Verification items for the finished model (mm, model axes). A direction names the side the tool comes from. Round coordinates to 2 decimals unless told otherwise and drop trailing zeros. Write each loop counter-clockwise with the first axis right and the second up, starting at its lowest first coordinate (ties: lowest second). Pieces come first, ordered by that corner, then holes.
from build123d import *
from build123d.topology import SkipClean

# Parameters (mm, degrees)
CUT_EXTRUDE1_DEPTH      = 35
CUT_EXTRUDE1_DEPTH_BACK = 35
SKETCH2_OUTSIDE_W       = 96.248
SKETCH2_OUTSIDE_H       = 96.248
BOSS_EXTRUDE1_DEPTH     = 36
SKETCH4_R               = 3.5
CUT_EXTRUDE2_DEPTH      = 5
LPATTERN1_COUNT         = 2
LPATTERN1_PITCH         = 35
BOSS_EXTRUDE2_DEPTH     = 50
BOSS_EXTRUDE6_DEPTH     = 15
SKETCH10_R              = 25
BOSS_EXTRUDE7_DEPTH     = 2
SKETCH11_R              = 3.5
BOSS_EXTRUDE8_DEPTH     = 5


with BuildPart() as part:
    # Sketch1 → Revolve2 (revolve)
    with BuildSketch(Plane(origin=(0, 0, 0), x_dir=(1, 0, 0), z_dir=(0, 1, 0))):
        with BuildLine():
            Line((0, 35), (0, -35))
            ThreePointArc((0, -35), (35, 0), (0, 35))
        make_face()
    revolve(axis=Axis((0, 0, -35), (0, 0, 1)))

    # Sketch2 outside → Cut-Extrude1 (cut, two sides: drawn at the far end of the back side and taken through both)
    with SkipClean():  # the faces are left unmerged after this step: merging them gives an invalid solid
        with BuildSketch(Plane(origin=(0, 0, 0), x_dir=(1, 0, 0), z_dir=(0, 1, 0)).offset(-CUT_EXTRUDE1_DEPTH_BACK)):
            Rectangle(SKETCH2_OUTSIDE_W, SKETCH2_OUTSIDE_H)
            with BuildLine():
                Line((-20, -28.722813233), (-20, 28.722813233))
                ThreePointArc((-20, 28.722813233), (0, 35), (20, 28.722813233))
                Line((20, 28.722813233), (20, -28.722813233))
                ThreePointArc((20, -28.722813233), (0, -35), (-20, -28.722813233))
            make_face(mode=Mode.SUBTRACT)
        extrude(amount=CUT_EXTRUDE1_DEPTH + CUT_EXTRUDE1_DEPTH_BACK, mode=Mode.SUBTRACT)

    # Sketch3 → Boss-Extrude1 (add)
    with BuildSketch(Plane(origin=(0, 0, 0), x_dir=(1, 0, 0), z_dir=(0, 1, 0))):
        with BuildLine():
            Line((-20, 15), (-20, -15))
            ThreePointArc((-20, -15), (0, -25), (20, -15))
            Line((20, -15), (20, 15))
            ThreePointArc((20, 15), (0, 25), (-20, 15))
        make_face()
    extrude(amount=BOSS_EXTRUDE1_DEPTH)

    # Sketch4 → Cut-Extrude2 (cut)
    with BuildSketch(Plane.ZY.offset(20)):
        Circle(SKETCH4_R)
    cut_extrude2 = extrude(amount=-CUT_EXTRUDE2_DEPTH, mode=Mode.SUBTRACT)

    # LPattern1: Cut-Extrude2 ×2
    with Locations(*[(i * LPATTERN1_PITCH, 0, 0) for i in range(1, LPATTERN1_COUNT)]):
        add(cut_extrude2, mode=Mode.SUBTRACT)

    # Sketch5 → Boss-Extrude2 (add)
    with BuildSketch(Plane(origin=(0, 36, 0), x_dir=(1, 0, 0), z_dir=(0, 1, 0))):
        with BuildLine():
            Line((-20, 15), (-20, 11.357816692))
            ThreePointArc((-20, 11.357816692), (-23, 0), (-20, -11.357816692))
            Line((-20, -11.357816692), (-20, -15))
            ThreePointArc((-20, -15), (0, -25), (20, -15))
            Line((20, -15), (20, -11.357816692))
            ThreePointArc((20, -11.357816692), (23, 0), (20, 11.357816692))
            Line((20, 11.357816692), (20, 15))
            ThreePointArc((20, 15), (0, 25), (-20, 15))
        make_face()
    extrude(amount=BOSS_EXTRUDE2_DEPTH)

    # Sketch9 → Boss-Extrude6 (add)
    with BuildSketch(Plane(origin=(0, 86, 0), x_dir=(1, 0, 0), z_dir=(0, 1, 0))):
        with BuildLine():
            Line((20, 11.357816692), (20, 15))
            ThreePointArc((20, 15), (0, 25), (-20, 15))
            Line((-20, 15), (-20, 11.357816692))
            ThreePointArc((-20, 11.357816692), (-23, 0), (-20, -11.357816692))
            Line((-20, -11.357816692), (-20, -15))
            ThreePointArc((-20, -15), (0, -25), (20, -15))
            Line((20, -15), (20, -11.357816692))
            ThreePointArc((20, -11.357816692), (23, 0), (20, 11.357816692))
        make_face()
    extrude(amount=BOSS_EXTRUDE6_DEPTH)

    # Sketch10 → Boss-Extrude7 (add)
    with BuildSketch(Plane(origin=(0, 101, 0), x_dir=(1, 0, 0), z_dir=(0, 1, 0))):
        with Locations(Location((0, 0, 0), (0, 0, 36.869897646))):
            Circle(SKETCH10_R)
    extrude(amount=BOSS_EXTRUDE7_DEPTH)

    # Sketch11 → Boss-Extrude8 (add)
    with BuildSketch(Plane(origin=(0, 103, 0), x_dir=(1, 0, 0), z_dir=(0, 1, 0))):
        with Locations(Location((0, 0, 0), (0, 0, 270))):
            Circle(SKETCH11_R)
    extrude(amount=BOSS_EXTRUDE8_DEPTH)


solid = part.part
Q1. Sectioned sample at A-A (x = 0). Enter the section's corners in (y, z), plus the area to 3 significant figures.
Recorded:
outline: (24.49, -25) - (103, -25) - (103, -3.5) - (108, -3.5) - (108, 3.5) - (103, 3.5) - (103, 25) - (24.49, 25) arc R35 ccw (long way) to start
area: 7,450 mm2
Q2. Depth check by flat-ended pin: P1, Ø4, axis at x = -14.5, y = -13.5, coming from the -Z side; P2, Ø3.5, axis at y = -0.5, z = 0.5, coming from the +X side; P3, Ø25, axis at x = 0.5, z = 7, coming from the +Y side; P4, Ø1, axis at x = 4, y = 19, coming from the -Z side. Enter the tip coordinate at first touch or a pass-through.
Recorded:
P1: stops at z = -30.13
P2: stops at x = 15
P3: stops at y = 108
P4: stops at z = -29.45
Q3. Sectioned sample at C-C (y = 74.5). Enter the section's corners in (x, z), plus the area to 3 significant figures.
Recorded:
outline: (-20, -15) arc R25 ccw to (20, -15) - (20, -11.36) arc R23 ccw to (20, 11.36) - (20, 15) arc R25 ccw to (-20, 15) - (-20, 11.36) arc R23 ccw to (-20, -11.36) - close
area: 1,850 mm2
Q4. Material ranges on line 1 along Y through (x, z) = (18.35, 0); line 2 along Y through (x, z) = (16.5, 0); line 3 along X through (y, z) = (12, -5.5), recorded low to high.
Recorded:
line 1: y = -29.8 to -3.5, 3.5 to 103
line 2: y = -30.87 to -3.5, 3.5 to 103
line 3: x = -20 to 20
Q5. Sectioned sample at D-D (y = 0). Enter the section's corners in (x, z).
Recorded:
outline: (-20, -28.72) arc R35 ccw to (20, -28.72) - (20, -3.5) - (15, -3.5) - (15, 3.5) - (20, 3.5) - (20, 28.72) arc R35 ccw to (-20, 28.72) - (-20, 3.5) - (-15, 3.5) - (-15, -3.5) - (-20, -3.5) - close
Q6. Sectioned sample at B-B (z = 0). Enter the section's corners in (x, y), plus the area to 3 significant figures.
Recorded:
outline: (-25, 101) - (-23, 101) - (-23, 36) - (-20, 36) - (-20, 3.5) - (-15, 3.5) - (-15, -3.5) - (-20, -3.5) - (-20, -28.72) arc R35 ccw to (20, -28.72) - (20, -3.5) - (15, -3.5) - (15, 3.5) - (20, 3.5) - (20, 36) - (23, 36) - (23, 101) - (25, 101) - (25, 103) - (3.5, 103) - (3.5, 108) - (-3.5, 108) - (-3.5, 103) - (-25, 103) - close
area: 5,810 mm2
Q7. Tool access check on faces 1 (the flat face through (21, 36, 0)), 2 (the flat face through (-23.3, 101, 0.2)), 3 (the cylindrical face through (17.465, -1.341, 3.233)). Record the directions out of +Z, -Z, +X, -X, +Y, -Y that give a thin tool (end or side, any length) a straight path to the whole face; none if there is none.
Recorded:
face 1: +Z, -Z, +X, -Y
face 2: -X, -Y
face 3: +X
Q8. Release check for a two-part mould opening along Y. For faces 4 (the flat face through (15, 0, 0)), 5 (the flat face through (23.133, 101, 0.914)), 6 (the cylindrical face through (-3.417, 105.465, -0.759)) record: released by +Y, released by -Y, zero draft, split by the parting line, or undercut.
Recorded:
face 4: undercut
face 5: released by -Y
face 6: zero draft
